from build123d import *

# Parameters (mm, degrees)
F1_DEPTH = 10
F3_R     = 14
F4_DEPTH = 5
F2_R     = 2
F5_DEPTH = 40
F7_DEPTH = 4


with BuildPart() as f1:
    # F0 (on Front) → F1 (new body)
    with BuildSketch(Plane.XZ):
        with BuildLine():
            ThreePointArc((10.115177, -5.84), (11.282014, -3.023006), (11.68, 0))
            ThreePointArc((11.68, 0), (11.679631, 0.092805), (11.678525, 0.185604))
            ThreePointArc((11.678525, 0.185604), (11.257638, 3.112553), (10.115177, 5.84))
            ThreePointArc((10.115177, 5.84), (8.193124, 8.324369), (5.678525, 10.206701))
            ThreePointArc((5.678525, 10.206701), (2.933269, 11.305677), (0, 11.68))
            ThreePointArc((0, 11.68), (-3.112553, 11.257638), (-6, 10.021098))
            ThreePointArc((-6, 10.021098), (-8.324369, 8.193124), (-10.115177, 5.84))
            ThreePointArc((-10.115177, 5.84), (-11.305677, 2.933269), (-11.678525, -0.185604))
            ThreePointArc((-11.678525, -0.185604), (-11.257638, -3.112553), (-10.115177, -5.84))
            ThreePointArc((-10.115177, -5.84), (-8.193124, -8.324369), (-5.678525, -10.206701))
            ThreePointArc((-5.678525, -10.206701), (-2.933269, -11.305677), (0, -11.68))
            ThreePointArc((0, -11.68), (3.112553, -11.257638), (6, -10.021098))
            ThreePointArc((6, -10.021098), (8.324369, -8.193124), (10.115177, -5.84))
        make_face()
        with BuildLine():
            ThreePointArc((11.678525, 0.185604), (11.679631, 0.092805), (11.68, 0))
            ThreePointArc((11.68, 0), (11.282014, -3.023006), (10.115177, -5.84))
            Line((10.115177, -5.84), (11.01996, -6.362377))
            ThreePointArc((11.01996, -6.362377), (12.244829, -3.186001), (12.596117, 0.200187))
            Line((12.596117, 0.200187), (11.678525, 0.185604))
        make_face()
        with BuildLine():
            ThreePointArc((5.678525, 10.206701), (8.193124, 8.324369), (10.115177, 5.84))
            Line((10.115177, 5.84), (11.01996, 6.362377))
            ThreePointArc((11.01996, 6.362377), (8.881572, 9.011333), (6.124692, 11.00865))
            Line((6.124692, 11.00865), (5.678525, 10.206701))
        make_face()
        with BuildLine():
            Line((6.471425, -10.808464), (6, -10.021098))
            ThreePointArc((6, -10.021098), (3.112553, -11.257638), (0, -11.68))
            Line((0, -11.68), (0, -12.724753))
            ThreePointArc((0, -12.724753), (3.363257, -12.197333), (6.471425, -10.808464))
        make_face()
        with BuildLine():
            ThreePointArc((-6, 10.021098), (-3.112553, 11.257638), (0, 11.68))
            Line((0, 11.68), (0, 12.724753))
            ThreePointArc((0, 12.724753), (-3.363257, 12.197333), (-6.471425, 10.808464))
            Line((-6.471425, 10.808464), (-6, 10.021098))
        make_face()
        with BuildLine():
            Line((-6.124692, -11.00865), (-5.678525, -10.206701))
            ThreePointArc((-5.678525, -10.206701), (-8.193124, -8.324369), (-10.115177, -5.84))
            Line((-10.115177, -5.84), (-11.01996, -6.362377))
            ThreePointArc((-11.01996, -6.362377), (-8.881572, -9.011333), (-6.124692, -11.00865))
        make_face()
        with BuildLine():
            ThreePointArc((-11.678525, -0.185604), (-11.305677, 2.933269), (-10.115177, 5.84))
            Line((-10.115177, 5.84), (-11.01996, 6.362377))
            ThreePointArc((-11.01996, 6.362377), (-12.244829, 3.186001), (-12.596117, -0.200187))
            Line((-12.596117, -0.200187), (-11.678525, -0.185604))
        make_face()
    extrude(amount=F1_DEPTH)

    # F3 (on face) → F4 (join)
    with BuildSketch(Plane(origin=(0, 0, 0), x_dir=(-1, 0, 0), z_dir=(0, 1, 0))):
        Circle(F3_R)
    extrude(amount=F4_DEPTH)

    # F2 (on face) → F5 (cut)
    with BuildSketch(Plane.XZ.offset(10)):
        Circle(F2_R)
    extrude(amount=-F5_DEPTH, mode=Mode.SUBTRACT)

    # F6 (on face) → F7 (cut)
    with BuildSketch(Plane(origin=(0, 5, 0), x_dir=(-1, 0, 0), z_dir=(0, 1, 0))):
        Polygon((1.148891, 3.874711), (-2.781153, 2.932324), (-3.930043, -0.942387), (-1.148891, -3.874711), (2.781153, -2.932324), (3.930043, 0.942387), align=None)
    extrude(amount=-F7_DEPTH, mode=Mode.SUBTRACT)


solid = f1.part
Check sheet for the modelled part. Datum: model origin and axes. Units: mm. A direction names the side the tool comes from. Give positions to 0.01 mm unless a question says otherwise; leave off trailing zeros. Loops run counter-clockwise (first coordinate to the right, second up) from the corner with the lowest first, then second, coordinate; pieces in that order, holes last. Notation, with made-up numbers: M 13.25,-10.5 L 25.25,-10.5 A10 ccw 25.25,0.5 Z; hole C 24,19 d11. An arc over 180 degrees is marked long. Return JSON: item names as keys, results as strings. Group by question number.
1. Thickness scan on L1, parallel to Y at x = 12, z = -6.75; L2, parallel to X at y = 3.5, z = -1.75; L3, parallel to X at y = -4.5, z = 1.75. Record the ranges inside material, lowest first.
2. Tool access check on faces 4 (the cylindrical face through (3.32, -4.93, -12.21)), 5 (the flat face through (10.561, -4.93, -6.098)), 6 (the flat face through (2.559, 3.028, -2.388)). Record the directions out of +Z, -Z, +X, -X, +Y, -Y that give a thin tool (end or side, any length) a straight path to the whole face; none if there is none.
3. Go/stop test with flat-tipped pins: pin 1 (2.5 mm diameter, centred on x = 0, z = 0, fed in from -Y); pin 2 (1 mm diameter, centred on y = -3, z = 3.5, fed in from +X); pin 3 (3 mm diameter, centred on y = 2, z = -2, fed in from +X); pin 4 (1 mm diameter, centred on x = -8, y = 1, fed in from -Z). Record where each tip stops, or that it passes through.
4. Cross-section at A-A on y = 3.25. Record the boundary of the cut face in (x, z), plus the area to 3 significant figures.
5. Cross-section at B-B on y = -4.5. Record the boundary of the cut face in (x, z).
6. Cross-section at C-C on z = 9.25. Record the boundary of the cut face in (x, y), plus the area to 3 significant figures.
7. Cross-section at D-D on x = -9.75. Record the boundary of the cut face in (y, z).
8. Mould release check, pull along X, two halves, no side actions. Record for faces 1 (the flat face through (-10.561, -4.93, 6.098)), 2 (the cylindrical face through (-8.916, -4.93, -8.978)), 3 (the flat face through (0, -5, 12)): released by +X, released by -X, zero draft, split by the parting line, or undercut.
Return value:
{
 "1": {"L1": "0 to 5", "L2": "-13.89 to -3.13, 3.16 to 13.89", "L3": "-12.5 to -0.97, 0.97 to 11.55"},
 "2": {"face 4": "-Z, +X, -Y", "face 5": "-Z, -Y", "face 6": "+Y"},
 "3": {"pin 1": "through", "pin 2": "x = 11.29", "pin 3": "x = 13.99", "pin 4": "z = -11.82"},
 "4": {"outline": "C 0,0 d28; hole M -3.93,0.94 L -2.78,-2.93 L 1.15,-3.87 L 3.93,-0.94 L 2.78,2.93 L -1.15,3.87 Z", "area": "573 mm^2"},
 "5": {"outline": "M -12.6,-0.2 L -11.68,-0.19 A11.68 ccw -10.12,-5.84 L -11.02,-6.36 A12.9 ccw -6.12,-11.01 L -5.68,-10.21 A11.68 ccw 0,-11.68 L 0,-12.72 A12.9 ccw 6.47,-10.81 L 6,-10.02 A11.68 ccw 10.12,-5.84 L 11.02,-6.36 A12.9 ccw 12.6,0.2 L 11.68,0.19 A11.68 ccw 10.12,5.84 L 11.02,6.36 A12.9 ccw 6.12,11.01 L 5.68,10.21 A11.68 ccw 0,11.68 L 0,12.72 A12.9 ccw -6.47,10.81 L -6,10.02 A11.68 ccw -10.12,5.84 L -11.02,6.36 A12.9 ccw Z; hole C 0,0 d4"},
 "6": {"outline": "M -10.51,0 L -7.13,0 L -7.13,-10 L 8.62,-10 L 8.62,0 L 10.51,0 L 10.51,5 L -10.51,5 Z", "area": "263 mm^2"},
 "7": {"outline": "M -10,-8.1 L 0,-8.1 L 0,-10.05 L 5,-10.05 L 5,10.05 L 0,10.05 L 0,6.43 L -10,6.43 Z"},
 "8": {"face 1": "undercut", "face 2": "released by -X", "face 3": "released by +X"}
}
